Could you check a few things on this model? Use its own coordinates, in mm. Face numbers are marked on the shaded views. Round coordinates to 2 decimals unless told otherwise and drop trailing zeros. Loops run counter-clockwise (first coordinate to the right, second up) from the corner with the lowest first, then second, coordinate; pieces in that order, holes last. Notation, with made-up numbers: (49.25, 79) -> (103.25, 79) arc R35 cw to (103.25, 115) -> close; hole circle Ø10 at (2.5, 30). An arc over 180 degrees is marked (long way). One line per item, written item: value.
from build123d import *

# Parameters (mm, degrees)
SKETCH2_W           = 12
SKETCH2_H           = 7.1
CUT_EXTRUDE2_DEPTH  = 30
BOSS_EXTRUDE1_DEPTH = 40
SKETCH5_R           = 10.55
CUT_EXTRUDE3_DEPTH  = 86.931397056


with BuildPart() as part:
    # Sketch1 → Revolve2 (revolve)
    with BuildSketch(Plane(origin=(0, 0, 0), x_dir=(1, 0, 0), z_dir=(0, 1, 0))):
        Polygon((8.05, 0), (15.05, 0), (15.05, 80.5), (10.55, 80.5), (10.55, 5.95), (8.05, 5.95), align=None)
    revolve(axis=Axis((0, 0, 0), (0, 0, -1)))

    # Sketch2 → Cut-Extrude2 (cut)
    with BuildSketch(Plane(origin=(0, 0, 0), x_dir=(0, 0, -1), z_dir=(1, 0, 0))):
        with Locations((52.5, 0)):
            Rectangle(SKETCH2_W, SKETCH2_H)
    extrude(amount=CUT_EXTRUDE2_DEPTH, mode=Mode.SUBTRACT)

    # Sketch3 → Boss-Extrude1 (add)
    with BuildSketch(Plane(origin=(0, 0, 0), x_dir=(0, 0, -1), z_dir=(1, 0, 0))):
        Polygon((46.5, -2), (43.5, -2), (43.5, -6), (52.5, -6), (61.5, -6), (61.5, -2), (58.5, -2), (58.5, -3.55), (46.5, -3.55), align=None)
    extrude(amount=BOSS_EXTRUDE1_DEPTH)

    # Sketch5 → Cut-Extrude3 (cut, through all)
    with BuildSketch(Plane.XY.offset(-5.95)):
        Circle(SKETCH5_R)
    extrude(amount=-CUT_EXTRUDE3_DEPTH, mode=Mode.SUBTRACT)


solid = part.part
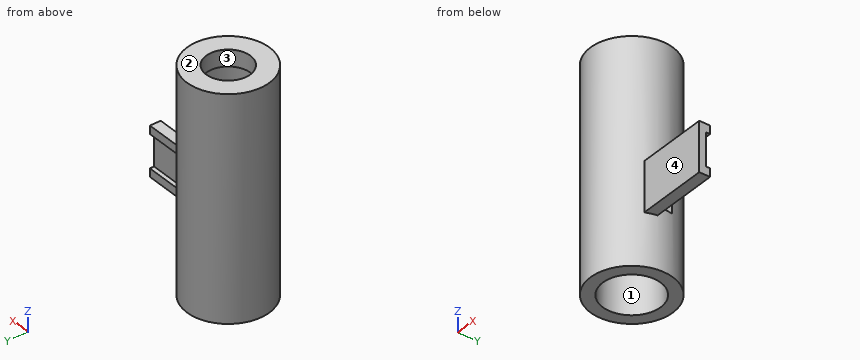
(1) If we section it at D-D, the plane x = 35.5: Please give me the cut outline in (y, z).
Recorded:
outline: (-6, -61.5) -> (-2, -61.5) -> (-2, -58.5) -> (-3.55, -58.5) -> (-3.55, -46.5) -> (-2, -46.5) -> (-2, -43.5) -> (-6, -43.5) -> close
(2) Thinking about a two-plate mould opening in Y: for the marked faces 1, 2, 3 and 4, which applies, released by +Y, released by -Y, zero draft, split by the parting line, or undercut?
Recorded:
face 1: undercut
face 2: zero draft
face 3: undercut
face 4: released by -Y
(3) If I drill on L1, parallel to X at y = 0, z = -1.4; L2, parallel to X at y = -0.5, z = -37; L3, parallel to Z at x = 8, y = -6, over which ranges is the centre line in solid material (lowest first)?
Recorded:
L1: -15.05 to -8.05, 8.05 to 15.05
L2: -15.04 to -10.54, 10.54 to 15.04
L3: -5.95 to 0
(4) I'm going to push flat-ended pins straight in: pin 1 Ø14.5 at (x, z) = (24, -56) entering from -Y; pin 2 Ø3.5 at (x, z) = (30, -45.5) entering from +Y; pin 3 Ø1.4 at (x, z) = (11.5, -52.5) entering from -Y; pin 4 Ø12 at (x, z) = (0.5, -66) entering from -Y. Where does each tip first touch, or does it pass through?
Recorded:
pin 1: y = -6
pin 2: y = -2
pin 3: y = -10.48
pin 4: y = -15.05
(5) If we section it at A-A, the plane x = 0: Please give me the cut outline in (y, z).
Recorded:
outline: (-15.05, -80.5) -> (-10.55, -80.5) -> (-10.55, -5.95) -> (-8.05, -5.95) -> (-8.05, 0) -> (-15.05, 0) -> close; (8.05, -5.95) -> (10.55, -5.95) -> (10.55, -80.5) -> (15.05, -80.5) -> (15.05, 0) -> (8.05, 0) -> close
(6) If we section it at B-B, the plane y = 0: Please give me the cut outline in (x, z).
Recorded:
outline: (-15.05, -80.5) -> (-10.55, -80.5) -> (-10.55, -5.95) -> (-8.05, -5.95) -> (-8.05, 0) -> (-15.05, 0) -> close; (8.05, -5.95) -> (10.55, -5.95) -> (10.55, -46.5) -> (15.05, -46.5) -> (15.05, 0) -> (8.05, 0) -> close; (10.55, -80.5) -> (15.05, -80.5) -> (15.05, -58.5) -> (10.55, -58.5) -> close
(7) If we section it at C-C, the plane y = 6: Please give me the cut outline in (x, z).
Recorded:
outline: (-13.8, -80.5) -> (-8.68, -80.5) -> (-8.68, -5.95) -> (-5.37, -5.95) -> (-5.37, 0) -> (-13.8, 0) -> close; (5.37, -5.95) -> (8.68, -5.95) -> (8.68, -80.5) -> (13.8, -80.5) -> (13.8, 0) -> (5.37, 0) -> close
